The drawing under review shows one solid part. Ordinate dimensions are in mm from its lowest x, y, z. A direction names the side the tool comes from. Give positions to 0.01 mm unless a question says otherwise; leave off trailing zeros. Loops run counter-clockwise (first coordinate to the right, second up) from the corner with the lowest first, then second, coordinate; pieces in that order, holes last. Notation, with made-up numbers: M 62,-5 L 90,-5 A20 ccw 90,29 Z; hole C 30.5,-22 d9. An arc over 180 degrees is marked long. Write item = value, one per line. Start each with the question number.
1. For the marked faces 1 and 2, list the 3-axis set-ups (+Z, -Z, +X, -X, +Y, -Y) from which the entire face can be reached by the end or side of a thin tool; tool diameter is ignored.
2. We need section A-A on z = 9. Give the boundary of the cut face in (x, y), then the cut area to 3 significant figures.
3. Draft analysis for pull direction X (two halves, no side actions). For the marked faces 3, 4, 5 and 6, state which applies: pulls with the +X half, pulls with the -X half, needs draft (parallel to the pull), parting line crosses it, or undercut.
4. We need section D-D on z = 30.5. Give the boundary of the cut face in (x, y).
5. Wall thickness on line 1 along X through (y, z) = (9.25, 13); line 2 along X through (y, z) = (1.5, 25); line 3 along Y through (x, z) = (67.5, 30): over which ranges is each line inside the solid? List them lowest first. Write a range as from..to.
6. For pin 1 (1.2 mm diameter, centred on x = 70, y = 3, fed in from -Z); pin 2 (2 mm diameter, centred on x = 81, z = 30, fed in from +Y), all flat-tipped, find the tip position at first contact; note any pin that passes through.
7. We need section B-B on x = 67. Give the boundary of the cut face in (y, z).
8. We need section C-C on y = 11.25. Give the boundary of the cut face in (x, z).
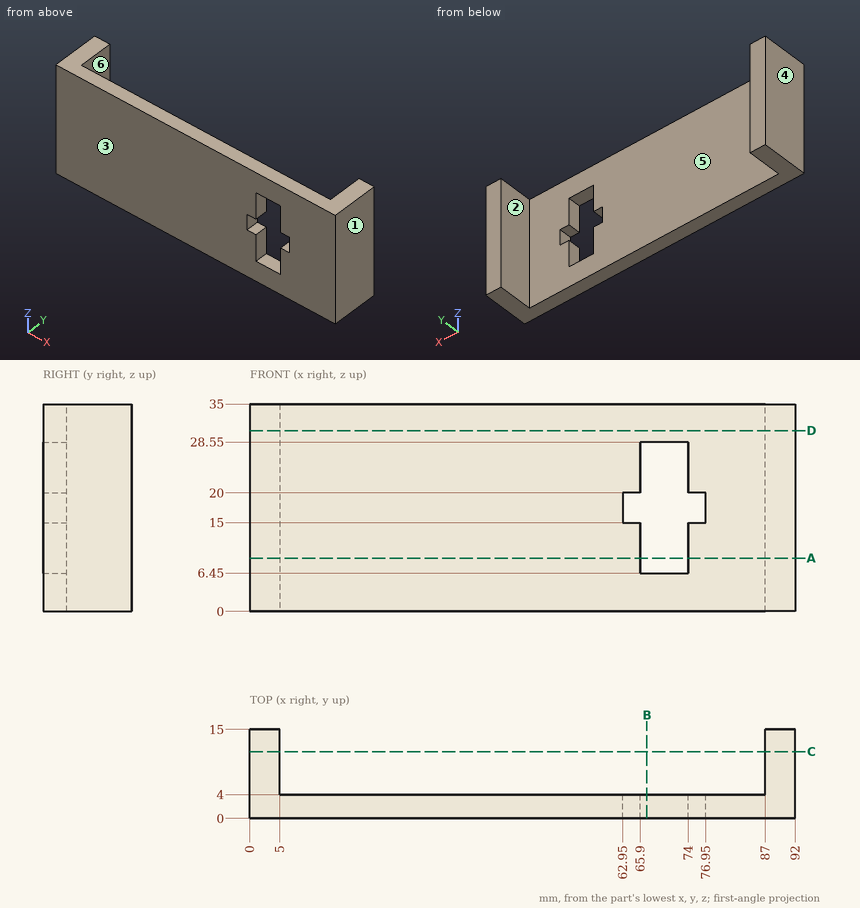
Final values:
q1.face_1 = +Z, -Z, +X, +Y, -Y
q1.face_2 = +Z, -Z, +Y
q2.outline = M 0,0 L 65.9,0 L 65.9,4 L 5,4 L 5,15 L 0,15 Z; M 74,0 L 92,0 L 92,15 L 87,15 L 87,4 L 74,4 Z
q2.area = 446 mm²
q3.face_3 = needs draft
q3.face_4 = pulls with the -X half
q3.face_5 = undercut
q3.face_6 = undercut
q4.outline = M 0,0 L 92,0 L 92,15 L 87,15 L 87,4 L 5,4 L 5,15 L 0,15 Z
q5.line_1 = 0..5, 87..92
q5.line_2 = 0..65.9, 74..92
q5.line_3 = 0..4
q6.pin_1 = 0
q6.pin_2 = 4
q7.outline = M 0,0 L 4,0 L 4,6.45 L 0,6.45 Z; M 0,28.55 L 4,28.55 L 4,35 L 0,35 Z
q8.outline = M 0,0 L 5,0 L 5,35 L 0,35 Z; M 87,0 L 92,0 L 92,35 L 87,35 Z
